from build123d import *

# Parameters (mm, degrees)
BOSS_EXTRUDE1_DEPTH  = 37.5
M3_CLEARANCE_HOLE1_D = 3.4
SKETCH4_R            = 12.5
CUT_EXTRUDE1_DEPTH   = 64.488187878
M5_CLEARANCE_HOLE1_D = 5.5
FILLET1_R            = 5


with BuildPart() as part:
    # Sketch1 → Boss-Extrude1 (new, symmetric)
    with BuildSketch(Plane(origin=(0, 0, 0), x_dir=(1, 0, 0), z_dir=(0, 1, 0))):
        Polygon((0, 0), (0, 20), (3.5, 20), (3.5, 3.5), (48.5, 3.5), (48.5, 0), align=None)
    extrude(amount=BOSS_EXTRUDE1_DEPTH, both=True)

    # M3 Clearance Hole1 (through all)
    with Locations(Plane(origin=(0, 0, -3.5), x_dir=(-1, 0, 0), z_dir=(0, 0, -1))):
        with Locations((-41.5, 15.5), (-10.5, 15.5), (-10.5, -15.5), (-41.5, -15.5)):
            Hole(M3_CLEARANCE_HOLE1_D / 2)

    # Sketch4 → Cut-Extrude1 (cut, through all)
    with BuildSketch(Plane(origin=(0, 0, -3.5), x_dir=(-1, 0, 0), z_dir=(0, 0, -1))):
        with Locations((-26, 0)):
            Circle(SKETCH4_R)
    extrude(amount=-CUT_EXTRUDE1_DEPTH, mode=Mode.SUBTRACT)

    # M5 Clearance Hole1 (through all)
    with Locations(Plane.ZY):
        with Locations((-10, 30.5), (-10, -30.5)):
            Hole(M5_CLEARANCE_HOLE1_D / 2)

    # Fillet1
    fillet1_edges = [part.edges().sort_by_distance(p)[0] for p in [
        (1.75, 37.5, -20),
        (1.75, -37.5, -20),
        (48.5, -37.5, -1.75),
        (48.5, 37.5, -1.75),
    ]]
    fillet(fillet1_edges, radius=FILLET1_R)


solid = part.part
For this review, take the finished solid that the model builds, in its own axes (mm). A direction names the side the tool comes from. Coordinates: 2 decimals unless noted, no trailing zeros. Order: outer loops, then holes, each group sorted by start corner. A loop starts at its lowest first (then second) coordinate and runs counter-clockwise, first axis right, second up. Notation, with made-up numbers: (3.25, 54) - (46.25, 54) arc R20 cw to (46.25, 77) - close; hole circle Ø4 at (-30, 57.5). An arc over 180 degrees is marked (long way). Answer as CSV lines item,"result". Start each with the question number.
1) Insertion check: P1, Ø8, axis at x = 32.5, y = 15.5, coming from the -Z side; P2, Ø9, axis at y = 30.5, z = -10, coming from the +X side; P3, Ø10, axis at x = 28.5, y = 6, coming from the -Z side. Each pin has a flat end and moves straight along its axis. Give the tip position at first contact, or say it passes through.
2) Add section C-C (y = 15.5). State the section outline as (x, z) points.
3) Machinability: for faces 5 (the cylindrical face through (11.3, 14, -1.7)), 6 (the flat face through (16, 9, -3.5)), which of the approach directions +Z, -Z, +X, -X, +Y, -Y give a long, thin tool a straight path to every point of the face, cutting with its end or side? Answer none if there is none.
4) Draft analysis for pull direction Z (two halves, no side actions). For faces 1 (the flat face through (14, 9, 0)), 2 (the flat face through (2, 0, -20)), 3 (the flat face through (48.5, 0, -2)), 4 (the cylindrical face through (1.77, 32.82, -11.48)), state which applies: +Z half, -Z half, draft (parallel to the pull), parting line (faces both ways), or undercut.
5) Add section D-D (y = -30.5). State the section outline as (x, z) points, then the cut area to 3 significant figures.
6) Add section B-B (x = 10.5). State the section outline as (y, z) points, then the cut area to 3 significant figures.
7) To check wall thickness, follow line 1 along Y through (x, z) = (41.5, -1); line 2 along Y through (x, z) = (0.75, -10); line 3 along Z through (x, y) = (42.5, 3). State the ranges of each line that lie inside material, in increasing order. Write a range as [from, to].
8) Add section A-A (z = -10). State the section outline as (x, y) points, then the cut area to 3 significant figures.
Result:
1,P1,"z = -3.5"
1,P2,"x = 3.5"
1,P3,"through"
2,outline,"(0, -20) - (3.5, -20) - (3.5, -3.5) - (8.8, -3.5) - (8.8, 0) - (0, 0) - close; (12.2, -3.5) - (39.8, -3.5) - (39.8, 0) - (12.2, 0) - close; (43.2, -3.5) - (48.5, -3.5) - (48.5, 0) - (43.2, 0) - close"
3,face 5,"+Z, -Z"
3,face 6,"-Z, +X, +Y, -Y"
4,face 1,"+Z half"
4,face 2,"-Z half"
4,face 3,"draft"
4,face 4,"undercut"
5,outline,"(0, -20) - (3.5, -20) - (3.5, -12.75) - (0, -12.75) - close; (0, -7.25) - (3.5, -7.25) - (3.5, -3.5) - (48.5, -3.5) - (48.5, 0) - (0, 0) - close"
5,area,"208 mm^2"
6,outline,"(-37.5, -3.5) - (-17.2, -3.5) - (-17.2, 0) - (-37.5, 0) - close; (-13.8, -3.5) - (13.8, -3.5) - (13.8, 0) - (-13.8, 0) - close; (17.2, -3.5) - (37.5, -3.5) - (37.5, 0) - (17.2, 0) - close"
6,area,"239 mm^2"
7,line 1,"[-37.5, -17.2], [-13.8, 13.8], [17.2, 37.5]"
7,line 2,"[-37.5, -33.25], [-27.75, 27.75], [33.25, 37.5]"
7,line 3,"[-3.5, 0]"
8,outline,"(0, -37.5) - (3.5, -37.5) - (3.5, -33.25) - (0, -33.25) - close; (0, -27.75) - (3.5, -27.75) - (3.5, 27.75) - (0, 27.75) - close; (0, 33.25) - (3.5, 33.25) - (3.5, 37.5) - (0, 37.5) - close"
8,area,"224 mm^2"
